Can you work these out from the model? Positions are in its coordinate system, mm. A direction names the side the tool comes from. Give positions to 0.01 mm unless a question says otherwise; leave off trailing zeros. Loops run counter-clockwise (first coordinate to the right, second up) from the corner with the lowest first, then second, coordinate; pieces in that order, holes last. Notation, with made-up numbers: (-39, -21.75) - (-4, -21.75) arc R19 ccw to (-4, 11.25) - close; hole circle Ø4 at (87.5, 84.25). An arc over 180 degrees is marked (long way). Use a Markdown table: item, result. Add a question column.
Autodesk Inventor part; units mm, degrees
ref_plane "YZ Plane" through (0, 0, 0) normal (1, 0, 0) x (0, 1, 0)
ref_plane "XZ Plane" through (0, 0, 0) normal (0, 1, 0) x (-1, 0, 0)
ref_plane "XY Plane" through (0, 0, 0) normal (0, 0, 1) x (1, 0, 0)
sketch "Sketch1" plane through (0, 0, 0) normal (0, 1, 0) x (-1, 0, 0)
  circle A0 centre (0, 0) radius 1.5
  dimension "d0" = 3
extrude "Extrusion1" add sketch "Sketch1" along normal blind 25
sketch "Sketch2" plane through (0, 0, 0) normal (0, -1, 0) x (1, 0, 0)
  circle A0 centre (0, 0) radius 2.5
  dimension "d3" = 5
extrude "Extrusion2" add sketch "Sketch2" along normal blind 2
chamfer "Chamfer1" distance 0.5 angle 45 1 edges at (1.5, 25, 0)
properties part number "M3x25Bolt"
1. Suppose I cut it at C-C (y = 13). List the corners of the cut face in (x, z) for me, and give its area (3 significant figures).
2. On a 3-axis mill with a long thin cutter (end or side, diameter ignored), from which of +Z, -Z, +X, -X, +Y, -Y can I reach the whole of each face in a straight line? I mean faces 1 (the face through (1.5, 12.08, -0.07)), 2 (the face through (0, 25, 0)). Say none if no direction works.
3. Suppose I cut it at A-A (x = 0). List the corners of the cut face in (y, z) for me, and give its area (4 significant figures).
4. Please list where these lines run through material, in increasing order: line 1 along Y through (x, z) = (-0.1, 1.9); line 2 along Z through (x, y) = (0, 15.75); line 3 along Z through (x, y) = (1.25, 13). Write a range as [from, to].
5. Suppose I cut it at B-B (z = 0). List the corners of the cut face in (x, y) for me, and give its area (4 significant figures).
6. Will these pins go through, and if not, where does the flat tip stop? P1, Ø1, axis at y = 18.5, z = 1.5, coming from the -X side; P2, Ø2, axis at x = 2, z = -0.5, coming from the +Y side; P3, Ø1.5, axis at y = 2.5, z = -2, coming from the -X side.
Results below:
| question | item | result |
|---|---|---|
| 1 | outline | circle Ø3 at (0, 0) |
| 1 | area | 7.07 mm² |
| 2 | face 1 | +Y |
| 2 | face 2 | +Z, -Z, +X, -X, +Y |
| 3 | outline | (-2, -2.5) - (0, -2.5) - (0, -1.5) - (24.5, -1.5) - (25, -1) - (25, 1) - (24.5, 1.5) - (0, 1.5) - (0, 2.5) - (-2, 2.5) - close |
| 3 | area | 84.75 mm² |
| 4 | line 1 | [-2, 0] |
| 4 | line 2 | [-1.5, 1.5] |
| 4 | line 3 | [-0.83, 0.83] |
| 5 | outline | (-2.5, -2) - (2.5, -2) - (2.5, 0) - (1.5, 0) - (1.5, 24.5) - (1, 25) - (-1, 25) - (-1.5, 24.5) - (-1.5, 0) - (-2.5, 0) - close |
| 5 | area | 84.75 mm² |
| 6 | P1 | x = -1.12 |
| 6 | P2 | y = 24.94 |
| 6 | P3 | x = -0.83 |
